Geometry: final body of the model. Coordinates: model frame, mm. A direction names the side the tool comes from. Give positions to 0.01 mm unless a question says otherwise; leave off trailing zeros. Loops run counter-clockwise (first coordinate to the right, second up) from the corner with the lowest first, then second, coordinate; pieces in that order, holes last. Notation, with made-up numbers: (10.5, 35) -> (69.5, 35) arc R16 cw to (69.5, 66) -> close; hole circle Ø8 at (54.5, 57). An arc over 180 degrees is marked (long way). One line per item, written item: value. Start each with the question number.
from build123d import *

# Parameters (mm, degrees)
SKETCH1_W           = 18
SKETCH1_H           = 40
BOSS_EXTRUDE1_DEPTH = 10
SKETCH3_W           = 5.5
SKETCH3_H           = 40
BOSS_EXTRUDE5_DEPTH = 2.5
SKETCH2_R           = 2.8
CUT_EXTRUDE1_DEPTH  = 13.5
SKETCH4_R           = 4.5
CUT_EXTRUDE2_DEPTH  = 5
SKETCH5_R           = 1.6
CUT_EXTRUDE3_DEPTH  = 13.5
SKETCH6_W           = 6
SKETCH6_H           = 2.5
CUT_EXTRUDE4_DEPTH  = 8


with BuildPart() as part:
    # Sketch1 → Boss-Extrude1 (new body)
    with BuildSketch(Plane(origin=(0, 0, 0), x_dir=(1, 0, 0), z_dir=(0, 1, 0))):
        with Locations((8.30324178, 20)):
            Rectangle(SKETCH1_W, SKETCH1_H)
    extrude(amount=BOSS_EXTRUDE1_DEPTH)

    # Sketch3 → Boss-Extrude5 (add)
    with BuildSketch(Plane.XZ):
        with Locations((8.30324178, -20)):
            Rectangle(SKETCH3_W, SKETCH3_H)
    extrude(amount=BOSS_EXTRUDE5_DEPTH)

    # Sketch2 → Cut-Extrude1 (cut, through all)
    with BuildSketch(Plane(origin=(0, 10, 0), x_dir=(1, 0, 0), z_dir=(0, 1, 0))):
        with Locations((8.30324178, 8)):
            Circle(SKETCH2_R)
    extrude(amount=-CUT_EXTRUDE1_DEPTH, mode=Mode.SUBTRACT)

    # Sketch4 → Cut-Extrude2 (cut)
    with BuildSketch(Plane(origin=(0, 10, 0), x_dir=(1, 0, 0), z_dir=(0, 1, 0))):
        with Locations((8.30324178, 8)):
            Circle(SKETCH4_R)
    extrude(amount=-CUT_EXTRUDE2_DEPTH, mode=Mode.SUBTRACT)

    # Sketch5 → Cut-Extrude3 (cut, through all)
    with BuildSketch(Plane(origin=(0, 10, 0), x_dir=(1, 0, 0), z_dir=(0, 1, 0))):
        with Locations((13.30324178, 16)):
            Circle(SKETCH5_R)
        with Locations((13.30324178, 35)):
            Circle(SKETCH5_R)
    extrude(amount=-CUT_EXTRUDE3_DEPTH, mode=Mode.SUBTRACT)

    # Sketch6 → Cut-Extrude4 (cut)
    with BuildSketch(Plane(origin=(17.30324178, 0, 0), x_dir=(0, 0, -1), z_dir=(1, 0, 0))):
        with Locations((16, 5.75)):
            Rectangle(SKETCH6_W, SKETCH6_H)
        with Locations((35, 5.75)):
            Rectangle(SKETCH6_W, SKETCH6_H)
    extrude(amount=-CUT_EXTRUDE4_DEPTH, mode=Mode.SUBTRACT)


solid = part.part
Item 1: Section A-A, the plane x = 10.25. Output: boundary loops of the cut face in (y, z).
Item 2: Pin query (flat end, axial travel): pin 1 (0.8 mm diameter, centred on y = -2, z = -30, fed in from -X); pin 2 (3 mm diameter, centred on x = 14, z = -26, fed in from -Y); pin 3 (0.8 mm diameter, centred on y = -1, z = -20, fed in from +X); pin 4 (3 mm diameter, centred on x = 13.3, z = -16, fed in from -Y). Return the tip coordinate at first contact, or that it passes through.
Item 3: Mould query, pull axis X, two halves, no side actions, for faces 6 (the face through (12.956, 8.521, -33.438)), 7 (the face through (9.303, 6, -16)), 8 (the face through (5.553, -1, -4)). Classes: pulls with the +X half, pulls with the -X half, needs draft (parallel to the pull), parting line crosses it, or undercut.
Item 4: Ray query, line 1 along Z through (x, y) = (11.5, 4.75); line 2 along Y through (x, z) = (12, -13.5); line 3 along X through (y, z) = (3.5, -16). Return the intervals inside material, ascending. Write a range as [from, to].
Item 5: Access query for faces 1 (the face through (11.053, -1, -4)), 2 (the face through (10.89, 1.3, -6.93)), 3 (the face through (13, 6, -38)), 4 (the face through (-0.697, 5, -20)), 5 (the face through (3.808, 7.535, -8.198)). Directions: +Z, -Z, +X, -X, +Y, -Y. A direction counts if a zero-diameter tool reaches every point of the face in a straight line with its end or side. Return the directions, or none.
Item 6: Section B-B, the plane y = 6.25. Output: boundary loops of the cut face in (x, z), then the cut area to 3 significant figures.
Item 7: Section C-C, the plane z = -8. Output: boundary loops of the cut face in (x, y), then the cut area to 3 significant figures.
Item 8: Section D-D, the plane y = -0.75. Output: boundary loops of the cut face in (x, z), then the cut area to 3 significant figures.
Geometry check:
1. outline: (-2.5, -40) -> (10, -40) -> (10, -12.06) -> (5, -12.06) -> (5, -10.01) -> (-2.5, -10.01) -> close; (-2.5, -5.99) -> (5, -5.99) -> (5, -3.94) -> (10, -3.94) -> (10, 0) -> (-2.5, 0) -> close; hole (4.5, -38) -> (7, -38) -> (7, -32) -> (4.5, -32) -> close; hole (4.5, -19) -> (7, -19) -> (7, -13) -> (4.5, -13) -> close
2. pin 1: stops at x = 5.55
2. pin 2: stops at y = 0
2. pin 3: stops at x = 11.05
2. pin 4: passes through
3. face 6: undercut
3. face 7: pulls with the +X half
3. face 8: pulls with the -X half
4. line 1: z = [-40, -38], [-32, -19], [-13, 0]
4. line 2: y = [0, 4.5], [7, 10]
4. line 3: x = [-0.7, 11.7], [14.9, 17.3]
5. face 1: +Z, -Z, +X, -Y
5. face 2: +Y, -Y
5. face 3: +X
5. face 4: +Z, -Z, -X, +Y, -Y
5. face 5: +Y
6. outline: (-0.7, -40) -> (17.3, -40) -> (17.3, -38) -> (9.3, -38) -> (9.3, -32) -> (17.3, -32) -> (17.3, -19) -> (9.3, -19) -> (9.3, -13) -> (17.3, -13) -> (17.3, 0) -> (-0.7, 0) -> close; hole circle Ø9 at (8.3, -8)
6. area: 560 mm2
7. outline: (-0.7, 0) -> (5.5, 0) -> (5.5, 5) -> (3.8, 5) -> (3.8, 10) -> (-0.7, 10) -> close; (11.1, 0) -> (17.3, 0) -> (17.3, 10) -> (12.8, 10) -> (12.8, 5) -> (11.1, 5) -> close
7. area: 107 mm2
8. outline: (5.55, -40) -> (11.05, -40) -> (11.05, -8.53) arc R2.8 cw to (5.55, -8.53) -> close; (5.55, -7.47) arc R2.8 cw to (11.05, -7.47) -> (11.05, 0) -> (5.55, 0) -> close
8. area: 195 mm2
